```python
from build123d import *

# Parameters (mm, degrees)
SKETCH1_R           = 5.0038
BOSS_EXTRUDE1_DEPTH = 1.6002
SKETCH2_R           = 2.38125
BOSS_EXTRUDE2_DEPTH = 17.78
FILLET1_R           = 2.54


with BuildPart() as part:
    # Sketch1 → Boss-Extrude1 (new body)
    with BuildSketch(Plane.XY):
        Circle(SKETCH1_R)
    extrude(amount=BOSS_EXTRUDE1_DEPTH)

    # Sketch2 → Boss-Extrude2 (add)
    with BuildSketch(Plane.XY):
        Circle(SKETCH2_R)
    extrude(amount=-BOSS_EXTRUDE2_DEPTH)

    # Fillet1
    # the kernel refuses this fillet: 2.54 mm, written as the material it takes off along each edge
    with BuildSketch(Plane(origin=(0, 0, 1.6002), x_dir=(1, 0, 0), z_dir=(0, -1, 0))) as fillet1_piece_1:
        with BuildLine():
            CenterArc((2.644059345, -2.54), FILLET1_R, 21.715617283, 68.284382717)
            Line((2.644059345, 0), (2.644059345, 0.0508))
            Line((2.644059345, 0.0508), (5.0038, 0.0508))
            Line((5.0038, 0.0508), (5.0546, 0))
            ThreePointArc((5.0546, 0), (5.0546, -0.8001), (5.050994813, -1.581404))
            Line((5.050994813, -1.581404), (5.0038, -1.6002))
        make_face()
    revolve(axis=Axis((0, 0, 1.6002), (0, 0, 1)), mode=Mode.SUBTRACT)


solid = part.part
```
Can you work these out from the model? Positions are in its coordinate system, mm. A direction names the side the tool comes from. Coordinates: 2 decimals unless noted, no trailing zeros. Loops run counter-clockwise (first coordinate to the right, second up) from the corner with the lowest first, then second, coordinate; pieces in that order, holes last. Notation, with made-up numbers: (2, -15) - (18, -15) arc R27 cw to (18, 5) - close; hole circle Ø7 at (68.25, -16.5). An arc over 180 degrees is marked (long way). Answer as CSV lines item,"result". Start each with the question number.
1) Suppose I cut it at A-A (x = 0). Please give me the cut outline in (y, z).
2) Suppose I cut it at D-D (z = 0.5). Please give me the cut outline in (x, y), plus the area to 3 significant figures.
3) Which directions (+Z, -Z, +X, -X, +Y, -Y) give clear straight access to the entire face, cutting with the end or side of a thin tool? Please do faces 1 (the cylindrical face through (-1.89, -1.45, -8.77)), 2 (the flat face through (0, 0, -17.78)).
4) Suppose I cut it at C-C (z = -8.25). Please give me the cut outline in (x, y), plus the area to 3 significant figures.
5) I need wall thicknesses on line 1 (Y direction, x = 0, z = -13.5); line 2 (X direction, y = -1, z = -16.5); line 3 (Z direction, x = -3.5, y = -3). Which ranges of each line are inside material? Lowest first, please. Write a range as from..to.
6) For pin 1 (3 mm diameter, centred on y = 0.5, z = -12.5, fed in from +X); pin 2 (6 mm diameter, centred on x = -1.5, y = 3, fed in from +Z); pin 3 (1.5 mm diameter, centred on x = 3, y = -1.5, fed in from -Z); pin 4 (6 mm diameter, centred on y = 1.5, z = -10.5, fed in from -X), each with a flat end and sliding along its axis, tell me the tip position at first contact or that it passes through.
Check result:
1,outline,"(-5, 0) - (-2.38, 0) - (-2.38, -17.78) - (2.38, -17.78) - (2.38, 0) - (5, 0) arc R2.54 ccw to (2.64, 1.6) - (-2.64, 1.6) arc R2.54 ccw to start"
2,outline,"circle Ø9.47 at (0, 0)"
2,area,"70.5 mm²"
3,face 1,"-Z"
3,face 2,"-Z, +X, -X, +Y, -Y"
4,outline,"circle Ø4.76 at (0, 0)"
4,area,"17.8 mm²"
5,line 1,"y = -2.38..2.38"
5,line 2,"x = -2.16..2.16"
5,line 3,"z = 0..0.67"
6,pin 1,"stops at x = 2.38"
6,pin 2,"stops at z = 1.6"
6,pin 3,"stops at z = 0"
6,pin 4,"stops at x = -2.38"
